Design review of the part built by this model. Coordinates are the model's own, in mm. A direction names the side the tool comes from. Round coordinates to 2 decimals unless told otherwise and drop trailing zeros. Loops run counter-clockwise (first coordinate to the right, second up) from the corner with the lowest first, then second, coordinate; pieces in that order, holes last. Notation, with made-up numbers: (88, 19.25) - (119, 19.25) arc R9 cw to (119, 24.25) - close; hole circle Ø10 at (-24, 3.5). An arc over 180 degrees is marked (long way). Answer as CSV lines item,"result". Start each with the question number.
(1) Consider section D-D (y = 4.5). Count the separate pieces of the cut face and the enclosed holes in it, and give its area (3 significant figures).
(2) Mouldability with a two-part tool opening along Z and no side actions: class faces 4 (the cylindrical face through (-11.076, 7.871, 27.993)), 5 (the cylindrical face through (-3.86, 7.83, -5.04)), 6 (the flat face through (-24, 15.875, 54)), 7 (the flat face through (0, 6, 57.15)) as released by +Z, released by -Z, zero draft, split by the parting line, or undercut.
(3) Consider section C-C (z = 7.5). Give the boundary of the cut face in (x, y) (3 decimals).
(4) Wall thickness on L1, parallel to X at y = 10.5, z = 50.8 (3 decimals); L2, parallel to Z at x = 0, y = 3.5 (3 decimals); L3, parallel to Z at x = -2, y = 6 (3 decimals): over which ranges is each line inside the solid? List them lowest first.
(5) For P1, Ø8, axis at x = -12.5, z = 18, coming from the +Y side, flat-tipped, find the tip position at first contact; note if it passes through.
(6) For faces 1 (the flat face through (0, 3.175, 36)), 2 (the flat face through (0, 12.7, 55)), 3 (the cylindrical face through (26.35, 7.83, 53.83)), list the 3-axis set-ups (+Z, -Z, +X, -X, +Y, -Y) from which the entire face can be reached by the end or side of a thin tool; tool diameter is ignored.
(7) Consider section B-B (z = 0). Give the boundary of the cut face in (x, y) (3 decimals).
(8) Consider section A-A (x = 0). Give the boundary of the cut face in (y, z) (3 decimals), and give its area (3 significant figures).
from build123d import *

# Parameters (mm, degrees)
BOSS_EXTRUDE1_DEPTH = 12.7
OUTSIDE_CIRLCES_R   = 9.525
OUTSIDE_CIRLCES_R_2 = 6.35
BOSS_EXTRUDE2_DEPTH = 15.875
SKETCH2_R           = 6.35
SKETCH2_R_2         = 3.175
CUT_EXTRUDE2_DEPTH  = 68.277043819
SHELL1_START        = 3.175
SHELL1_DEPTH        = 9.525
FILLET1_R           = 3.429


# Read off the part's stored shape, not the designer's step: Shell1
with BuildPart() as part:
    # Sketch1 → Boss-Extrude1 (new body)
    with BuildSketch(Plane(origin=(0, 0, 0), x_dir=(1, 0, 0), z_dir=(0, 1, 0))):
        with BuildLine():
            Line((-25.4, -57.15), (25.4, -57.15))
            ThreePointArc((25.4, -57.15), (31.415385717, -52.834117665), (29.253859008, -45.753192024))
            ThreePointArc((29.253859008, -45.753192024), (13.590190704, -25.845719106), (9.487062801, -0.849272876))
            ThreePointArc((9.487062801, -0.849272876), (0, 9.525), (-9.487062801, -0.849272876))
            ThreePointArc((-9.487062801, -0.849272876), (-13.590190704, -25.845719106), (-29.253859008, -45.753192024))
            ThreePointArc((-29.253859008, -45.753192024), (-31.415385717, -52.834117665), (-25.4, -57.15))
        make_face()
    extrude(amount=BOSS_EXTRUDE1_DEPTH)

    # Outside Cirlces → Boss-Extrude2 (add)
    with BuildSketch(Plane(origin=(0, 0, 0), x_dir=(1, 0, 0), z_dir=(0, 1, 0))):
        with Locations(Location((0, 0, 0), (0, 0, 354.884571445))):
            Circle(OUTSIDE_CIRLCES_R)
        with Locations(Location((25.4, -50.8, 0), (0, 0, 270))):
            Circle(OUTSIDE_CIRLCES_R_2)
        with Locations(Location((-25.4, -50.8, 0), (0, 0, 90))):
            Circle(OUTSIDE_CIRLCES_R_2)
    extrude(amount=BOSS_EXTRUDE2_DEPTH)

    # Sketch2 → Cut-Extrude2 (cut, through all)
    with BuildSketch(Plane(origin=(0, 0, 0), x_dir=(1, 0, 0), z_dir=(0, 1, 0))):
        with Locations(Location((0, 0, 0), (0, 0, 270))):
            Circle(SKETCH2_R)
        with Locations(Location((-25.4, -50.8, 0), (0, 0, 270))):
            Circle(SKETCH2_R_2)
        with Locations(Location((25.4, -50.8, 0), (0, 0, 270))):
            Circle(SKETCH2_R_2)
    extrude(amount=CUT_EXTRUDE2_DEPTH, mode=Mode.SUBTRACT)

    # Shell1 outline → Shell1 (cut)
    with BuildSketch(Plane(origin=(0, 0, 0), x_dir=(1, 0, 0), z_dir=(0, 1, 0)).offset(SHELL1_START)):
        with BuildLine():
            ThreePointArc((-23.245193613, -44.826783996), (-19.436053982, -48.61966794), (-19.900738686, -53.975))
            Line((-19.900738686, -53.975), (19.900738686, -53.975))
            ThreePointArc((19.900738686, -53.975), (19.436053982, -48.61966794), (23.245193613, -44.826783996))
            ThreePointArc((23.245193613, -44.826783996), (10.964919098, -27.751584466), (6.1431994, -7.279198179))
            ThreePointArc((6.1431994, -7.279198179), (0, -9.525), (-6.1431994, -7.279198179))
            ThreePointArc((-6.1431994, -7.279198179), (-10.964919098, -27.751584466), (-23.245193613, -44.826783996))
        make_face()
    extrude(amount=SHELL1_DEPTH, mode=Mode.SUBTRACT)

    # Fillet1
    fillet1_edges = [part.edges().sort_by_distance(p)[0] for p in [
        (-6.1431994, 7.9375, 7.279198179),
        (-19.900738686, 7.9375, 53.975),
        (23.245193613, 7.9375, 44.826783996),
        (6.1431994, 7.9375, 7.279198179),
        (-23.245193613, 7.9375, 44.826783996),
        (19.900738686, 7.9375, 53.975),
    ]]
    fillet(fillet1_edges, radius=FILLET1_R)


solid = part.part
Determined:
1,separate pieces,"1"
1,enclosed holes,"4"
1,area,"789 mm^2"
2,face 4,"undercut"
2,face 5,"undercut"
2,face 6,"zero draft"
2,face 7,"released by +Z"
3,outline,"(-9.329, 0) - (9.329, 0) - (9.329, 12.7) - (5.872, 12.7) - (5.872, 15.875) - (-5.872, 15.875) - (-5.872, 12.7) - (-9.329, 12.7) - close"
4,L1,"x = -31.75 to -28.575, -22.225 to -19.044, 19.044 to 22.225, 28.575 to 31.75"
4,L2,"z = -9.525 to -6.35, 6.35 to 9.525, 53.975 to 57.15"
4,L3,"z = -9.313 to -6.027, 6.027 to 9.313, 53.975 to 57.15"
5,P1,"stops at y = 12.7"
6,face 1,"+Y"
6,face 2,"+Z, +Y"
6,face 3,"+Y, -Y"
7,outline,"(-9.525, 0) - (-6.35, 0) - (-6.35, 15.875) - (-9.525, 15.875) - close; (6.35, 0) - (9.525, 0) - (9.525, 15.875) - (6.35, 15.875) - close"
8,outline,"(0, -9.525) - (15.875, -9.525) - (15.875, -6.35) - (0, -6.35) - close; (0, 6.35) - (15.875, 6.35) - (15.875, 9.525) - (3.175, 9.525) - (3.175, 53.975) - (12.7, 53.975) - (12.7, 57.15) - (0, 57.15) - close"
8,area,"282 mm^2"
